Can you work these out from the model? Positions are in its coordinate system, mm. Give positions to 0.01 mm unless a question says otherwise; leave off trailing zeros. Loops run counter-clockwise (first coordinate to the right, second up) from the corner with the lowest first, then second, coordinate; pieces in that order, holes last. Notation, with made-up numbers: (71, 68.25) - (107, 68.25) arc R5 cw to (107, 75.25) - close; hole circle Ø4 at (-32, -20.5). An arc over 180 degrees is marked (long way). Answer in a Markdown table with one row per item.
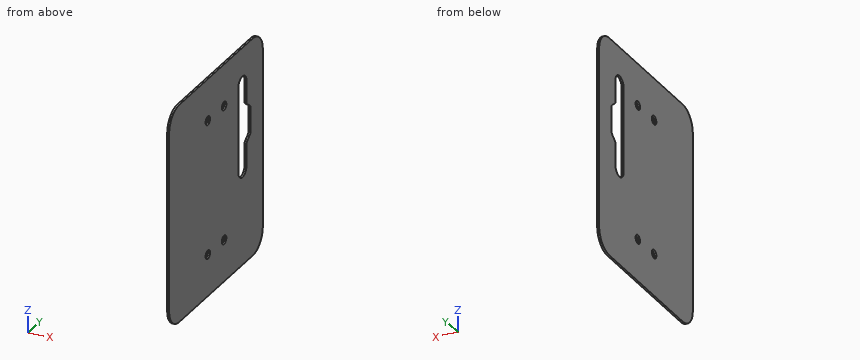
from build123d import *

# Parameters (mm, degrees)
SKETCH_1_R          = 1.1
EXTRUDE_1_DEPTH     = 0.5
CUT_EXTRUDE_1_DEPTH = 10
FILLET_1_R          = 1


with BuildPart() as part:
    # 草图1 → Extrude 1 (new body)
    with BuildSketch(Plane(origin=(0, 0, 0), x_dir=(0, 0, -1), z_dir=(1, 0, 0))):
        with BuildLine():
            Line((-23, 23), (23, 23))
            ThreePointArc((23, 23), (26.535533906, 21.535533906), (28, 18))
            Line((28, 18), (28, -18))
            ThreePointArc((28, -18), (26.535533906, -21.535533906), (23, -23))
            Line((23, -23), (-23, -23))
            ThreePointArc((-23, -23), (-26.535533906, -21.535533906), (-28, -18))
            Line((-28, -18), (-28, 18))
            ThreePointArc((-28, 18), (-26.535533906, 21.535533906), (-23, 23))
        make_face()
        with Locations((17.25, 4)):
            Circle(SKETCH_1_R, mode=Mode.SUBTRACT)
        with Locations((17.25, -4)):
            Circle(SKETCH_1_R, mode=Mode.SUBTRACT)
        with Locations((-17.25, -4)):
            Circle(SKETCH_1_R, mode=Mode.SUBTRACT)
        with Locations((-17.25, 4)):
            Circle(SKETCH_1_R, mode=Mode.SUBTRACT)
    extrude(amount=EXTRUDE_1_DEPTH)

    # 草图2 → 切除-拉伸1 (cut)
    with BuildSketch(Plane(origin=(0.5, 0, 0), x_dir=(0, 0, -1), z_dir=(1, 0, 0))):
        with BuildLine():
            Line((-18.6, 11), (3.4, 11))
            ThreePointArc((3.4, 11), (5.4, 13), (3.4, 15))
            Line((3.4, 15), (-18.6, 15))
            ThreePointArc((-18.6, 15), (-20.6, 13), (-18.6, 11))
        make_face()
        Polygon((-11.1, 17), (-12.6, 15), (-2.6, 15), (-4.1, 17), align=None)
    extrude(amount=-CUT_EXTRUDE_1_DEPTH, mode=Mode.SUBTRACT)

    # 圆角1
    fillet_1_edges = [part.edges().sort_by_distance(p)[0] for p in [
        (0.25, 15, 12.6),
        (0.25, 17, 11.1),
        (0.25, 17, 4.1),
        (0.25, 15, 2.6),
    ]]
    fillet(fillet_1_edges, radius=FILLET_1_R)


solid = part.part
Q1. For pin 1 (4 mm diameter, centred on y = -8.5, z = 6.5, fed in from -X), with a flat end and sliding along its axis, tell me the tip position at first contact or that it passes through.
Checked values:
| item | result |
|---|---|
| pin 1 | stops at x = 0 |
Q2. Imagine slicing it at B-B, the plane y = -4. Write out the boundary of the cut face in (x, z), and give its area (3 significant figures).
Checked values:
| item | result |
|---|---|
| outline | (0, -28) - (0.5, -28) - (0.5, -18.35) - (0, -18.35) - close; (0, -16.15) - (0.5, -16.15) - (0.5, 16.15) - (0, 16.15) - close; (0, 18.35) - (0.5, 18.35) - (0.5, 28) - (0, 28) - close |
| area | 25.8 mm² |
Q3. Imagine slicing it at D-D, the plane x = 0.1. Write out the boundary of the cut face in (y, z), and give its area (3 significant figures).
Checked values:
| item | result |
|---|---|
| outline | (-23, -23) arc R5 ccw to (-18, -28) - (18, -28) arc R5 ccw to (23, -23) - (23, 23) arc R5 ccw to (18, 28) - (-18, 28) arc R5 ccw to (-23, 23) - close; hole circle Ø2.2 at (-4, -17.25); hole circle Ø2.2 at (-4, 17.25); hole circle Ø2.2 at (4, -17.25); hole circle Ø2.2 at (4, 17.25); hole (11, -3.4) arc R2 ccw to (15, -3.4) - (15, 2.1) arc R1 cw to (15.4, 2.9) - (16.6, 3.8) arc R1 ccw to (17, 4.6) - (17, 10.6) arc R1 ccw to (16.6, 11.4) - (15.4, 12.3) arc R1 cw to (15, 13.1) - (15, 18.6) arc R2 ccw to (11, 18.6) - close |
| area | 2,420 mm² |
Q4. Imagine slicing it at A-A, the plane z = 17.25. Write out the boundary of the cut face in (x, y).
Checked values:
| item | result |
|---|---|
| outline | (0, -23) - (0.5, -23) - (0.5, -5.1) - (0, -5.1) - close; (0, -2.9) - (0.5, -2.9) - (0.5, 2.9) - (0, 2.9) - close; (0, 5.1) - (0.5, 5.1) - (0.5, 11) - (0, 11) - close; (0, 15) - (0.5, 15) - (0.5, 23) - (0, 23) - close |
Q5. If I drill on line 1 (Y direction, x = 0.2, z = -17.25); line 2 (Y direction, x = 0.1, z = 17.25); line 3 (Y direction, x = 0.25, z = 13), over which ranges is the centre line in solid material (lowest first)? Write a range as [from, to].
Checked values:
| item | result |
|---|---|
| line 1 | y = [-23, -5.1], [-2.9, 2.9], [5.1, 23] |
| line 2 | y = [-23, -5.1], [-2.9, 2.9], [5.1, 11], [15, 23] |
| line 3 | y = [-23, 11], [15.01, 23] |
Q6. Imagine slicing it at C-C, the plane z = 0.5. Write out the boundary of the cut face in (x, y).
Checked values:
| item | result |
|---|---|
| outline | (0, -23) - (0.5, -23) - (0.5, 11) - (0, 11) - close; (0, 15) - (0.5, 15) - (0.5, 23) - (0, 23) - close |
